Could you check a few things on this model? Use its own coordinates, in mm. A direction names the side the tool comes from. Give positions to 0.01 mm unless a question says otherwise; leave off trailing zeros. Write each loop counter-clockwise with the first axis right and the second up, starting at its lowest first coordinate (ties: lowest second). Pieces come first, ordered by that corner, then holes. Notation, with made-up numbers: M 70.5,57.5 L 129.5,57.5 A26 cw 129.5,82.5 Z; hole C -38,73.25 d11. An arc over 180 degrees is marked long. One line per item, written item: value.
```python
from build123d import *

# Parameters (mm, degrees)
SKETCH1_W                    = 482.6
SKETCH1_H                    = 381
BOSS_EXTRUDE1_DEPTH          = 0.9144
CONVERT_SOLID1_START         = -241.3
CONVERT_SOLID1_OUTLINE_W     = 0.6858
CONVERT_SOLID1_OUTLINE_H     = 381
CONVERT_SOLID1_DEPTH         = 482.6
EDGE_FLANGE1_STRIP_W         = 9.6012
EDGE_FLANGE1_STRIP_H         = 1.6002
EDGE_FLANGE1_STRIP_CUT_DEPTH = 381
EDGE_FLANGE1_DEPTH           = 381
EDGE_FLANGE2_STRIP_W         = 9.6012
EDGE_FLANGE2_STRIP_H         = 1.6002
EDGE_FLANGE2_STRIP_CUT_DEPTH = 381
EDGE_FLANGE2_DEPTH           = 381
EDGE_FLANGE3_STRIP_W         = 9.6012
EDGE_FLANGE3_STRIP_H         = 1.6002
EDGE_FLANGE3_STRIP_CUT_DEPTH = 381
EDGE_FLANGE3_DEPTH           = 381
EDGE_FLANGE4_STRIP_W         = 9.6012
EDGE_FLANGE4_STRIP_H         = 1.6002
EDGE_FLANGE4_STRIP_CUT_DEPTH = 381
EDGE_FLANGE4_DEPTH           = 381
EDGE_FLANGE5_STRIP_W         = 9.6012
EDGE_FLANGE5_STRIP_H         = 1.6002
EDGE_FLANGE5_STRIP_CUT_DEPTH = 381
EDGE_FLANGE5_DEPTH           = 381
SKETCH26_R                   = 3.2639
CUT_EXTRUDE2_DEPTH           = 2.54
SKETCH29_R                   = 3.2639
CUT_EXTRUDE4_DEPTH           = 310.870566463
SKETCH30_R                   = 3.2639
CUT_EXTRUDE5_DEPTH           = 2.54
SKETCH31_R                   = 3.19661248
CUT_EXTRUDE6_DEPTH           = 2.54
SKETCH32_R                   = 3.2639
CUT_EXTRUDE7_DEPTH           = 2.54


# Read off the part's stored shape, not the designer's step: Convert-Solid1
# Sheet-metal steps are written as plain solids
with BuildPart() as part:
    # Sketch1 → Boss-Extrude1 (new body)
    with BuildSketch(Plane(origin=(0, 0, 0), x_dir=(0, 0, -1), z_dir=(1, 0, 0))):
        Rectangle(SKETCH1_W, SKETCH1_H)
    extrude(amount=BOSS_EXTRUDE1_DEPTH)

    # Convert-Solid1 outline → Convert-Solid1 (add)
    with BuildSketch(Plane.XY.offset(CONVERT_SOLID1_START)):
        with Locations((-0.3429, 0)):
            Rectangle(CONVERT_SOLID1_OUTLINE_W, CONVERT_SOLID1_OUTLINE_H)
    extrude(amount=CONVERT_SOLID1_DEPTH)

    # Edge-Flange1 strip (across the edge) → Edge-Flange1 strip cut (cut)
    with BuildSketch(Plane(origin=(-0.6858, 190.5, -241.3), x_dir=(0, 0, 1), z_dir=(0, -1, 0))):
        with Locations((-3.2004, -0.8001)):
            Rectangle(EDGE_FLANGE1_STRIP_W, EDGE_FLANGE1_STRIP_H)
    extrude(amount=EDGE_FLANGE1_STRIP_CUT_DEPTH, mode=Mode.SUBTRACT)

    # Edge-Flange1 section (across the edge) → Edge-Flange1 (add)
    with BuildSketch(Plane(origin=(-0.6858, 190.5, -241.3), x_dir=(0, 0, 1), z_dir=(0, -1, 0))):
        with BuildLine():
            Line((-1.6002, 1.6002), (-1.6002, 23.7998))
            Line((-1.6002, 23.7998), (0, 23.7998))
            Line((0, 23.7998), (0, 1.6002))
            ThreePointArc((0, 1.6002), (0.468687729, 0.468687729), (1.6002, 0))
            Line((1.6002, 0), (1.6002, -1.6002))
            ThreePointArc((1.6002, -1.6002), (-0.662824543, -0.662824543), (-1.6002, 1.6002))
        make_face()
    extrude(amount=EDGE_FLANGE1_DEPTH)

    # Edge-Flange2 strip (across the edge) → Edge-Flange2 strip cut (cut)
    with BuildSketch(Plane(origin=(-24.4856, 190.5, -241.3), x_dir=(1, 0, 0), z_dir=(0, -1, 0))):
        with Locations((-3.2004, -0.8001)):
            Rectangle(EDGE_FLANGE2_STRIP_W, EDGE_FLANGE2_STRIP_H)
    extrude(amount=EDGE_FLANGE2_STRIP_CUT_DEPTH, mode=Mode.SUBTRACT)

    # Edge-Flange2 section (across the edge) → Edge-Flange2 (add)
    with BuildSketch(Plane(origin=(-24.4856, 190.5, -241.3), x_dir=(1, 0, 0), z_dir=(0, -1, 0))):
        with BuildLine():
            Line((-1.6002, 1.6002), (-1.6002, 23.7998))
            Line((-1.6002, 23.7998), (0, 23.7998))
            Line((0, 23.7998), (0, 1.6002))
            ThreePointArc((0, 1.6002), (0.468687729, 0.468687729), (1.6002, 0))
            Line((1.6002, 0), (1.6002, -1.6002))
            ThreePointArc((1.6002, -1.6002), (-0.662824543, -0.662824543), (-1.6002, 1.6002))
        make_face()
    extrude(amount=EDGE_FLANGE2_DEPTH)

    # Edge-Flange3 strip (across the edge) → Edge-Flange3 strip cut (cut)
    with BuildSketch(Plane(origin=(-0.6858, -190.5, 241.3), x_dir=(0, 0, -1), z_dir=(0, 1, 0))):
        with Locations((-3.2004, -0.8001)):
            Rectangle(EDGE_FLANGE3_STRIP_W, EDGE_FLANGE3_STRIP_H)
    extrude(amount=EDGE_FLANGE3_STRIP_CUT_DEPTH, mode=Mode.SUBTRACT)

    # Edge-Flange3 section (across the edge) → Edge-Flange3 (add)
    with BuildSketch(Plane(origin=(-0.6858, -190.5, 241.3), x_dir=(0, 0, -1), z_dir=(0, 1, 0))):
        with BuildLine():
            Line((-1.6002, 1.6002), (-1.6002, 23.7998))
            Line((-1.6002, 23.7998), (0, 23.7998))
            Line((0, 23.7998), (0, 1.6002))
            ThreePointArc((0, 1.6002), (0.468687729, 0.468687729), (1.6002, 0))
            Line((1.6002, 0), (1.6002, -1.6002))
            ThreePointArc((1.6002, -1.6002), (-0.662824543, -0.662824543), (-1.6002, 1.6002))
        make_face()
    extrude(amount=EDGE_FLANGE3_DEPTH)

    # Edge-Flange4 strip (across the edge) → Edge-Flange4 strip cut (cut)
    with BuildSketch(Plane(origin=(-24.4856, -190.5, 241.3), x_dir=(1, 0, 0), z_dir=(0, 1, 0))):
        with Locations((-3.2004, -0.8001)):
            Rectangle(EDGE_FLANGE4_STRIP_W, EDGE_FLANGE4_STRIP_H)
    extrude(amount=EDGE_FLANGE4_STRIP_CUT_DEPTH, mode=Mode.SUBTRACT)

    # Edge-Flange4 section (across the edge) → Edge-Flange4 (add)
    with BuildSketch(Plane(origin=(-24.4856, -190.5, 241.3), x_dir=(1, 0, 0), z_dir=(0, 1, 0))):
        with BuildLine():
            Line((-1.6002, 1.6002), (-1.6002, 23.7998))
            Line((-1.6002, 23.7998), (0, 23.7998))
            Line((0, 23.7998), (0, 1.6002))
            ThreePointArc((0, 1.6002), (0.468687729, 0.468687729), (1.6002, 0))
            Line((1.6002, 0), (1.6002, -1.6002))
            ThreePointArc((1.6002, -1.6002), (-0.662824543, -0.662824543), (-1.6002, 1.6002))
        make_face()
    extrude(amount=EDGE_FLANGE4_DEPTH)

    # Edge-Flange5 strip (across the edge) → Edge-Flange5 strip cut (cut)
    with BuildSketch(Plane(origin=(-26.0858, 190.5, 217.5002), x_dir=(0, 0, 1), z_dir=(0, -1, 0))):
        with Locations((-3.2004, -0.8001)):
            Rectangle(EDGE_FLANGE5_STRIP_W, EDGE_FLANGE5_STRIP_H)
    extrude(amount=EDGE_FLANGE5_STRIP_CUT_DEPTH, mode=Mode.SUBTRACT)

    # Edge-Flange5 section (across the edge) → Edge-Flange5 (add)
    with BuildSketch(Plane(origin=(-26.0858, 190.5, 217.5002), x_dir=(0, 0, 1), z_dir=(0, -1, 0))):
        with BuildLine():
            Line((-1.6002, 1.6002), (-1.6002, 23.7998))
            Line((-1.6002, 23.7998), (0, 23.7998))
            Line((0, 23.7998), (0, 1.6002))
            ThreePointArc((0, 1.6002), (0.468687729, 0.468687729), (1.6002, 0))
            Line((1.6002, 0), (1.6002, -1.6002))
            ThreePointArc((1.6002, -1.6002), (-0.662824543, -0.662824543), (-1.6002, 1.6002))
        make_face()
    extrude(amount=EDGE_FLANGE5_DEPTH)

    # Sketch26 → Cut-Extrude2 (cut)
    with BuildSketch(Plane(origin=(0, 0, 215.9), x_dir=(-1, 0, 0), z_dir=(0, 0, -1))):
        with Locations((39.41318, 152.4)):
            Circle(SKETCH26_R)
        with Locations((39.41318, 76.2)):
            Circle(SKETCH26_R)
        with Locations((39.41318, 0)):
            Circle(SKETCH26_R)
        with Locations((39.41318, -76.2)):
            Circle(SKETCH26_R)
        with Locations((39.41318, -152.4)):
            Circle(SKETCH26_R)
    extrude(amount=-CUT_EXTRUDE2_DEPTH, mode=Mode.SUBTRACT)

    # Sketch29 → Cut-Extrude4 (cut, through all)
    with BuildSketch(Plane.ZY.offset(26.0858)):
        with Locations((-228.6, 152.4)):
            Circle(SKETCH29_R)
        with Locations((-228.6, 76.2)):
            Circle(SKETCH29_R)
        with Locations((-228.6, 0)):
            Circle(SKETCH29_R)
        with Locations((-228.6, -76.2)):
            Circle(SKETCH29_R)
        with Locations((-228.6, -152.4)):
            Circle(SKETCH29_R)
    extrude(amount=-CUT_EXTRUDE4_DEPTH, mode=Mode.SUBTRACT)

    # Sketch30 → Cut-Extrude5 (cut)
    with BuildSketch(Plane.XY.offset(242.9002)):
        with Locations((-11.176, 152.4)):
            Circle(SKETCH30_R)
        with Locations((-11.176, 76.2)):
            Circle(SKETCH30_R)
        with Locations((-11.176, 0)):
            Circle(SKETCH30_R)
        with Locations((-11.176, -76.2)):
            Circle(SKETCH30_R)
        with Locations((-11.176, -152.4)):
            Circle(SKETCH30_R)
    extrude(amount=-CUT_EXTRUDE5_DEPTH, mode=Mode.SUBTRACT)

    # Sketch31 → Cut-Extrude6 (cut)
    with BuildSketch(Plane(origin=(0.9144, 0, 0), x_dir=(0, 0, -1), z_dir=(1, 0, 0))):
        with Locations((-217.5002, 178.689)):
            Circle(SKETCH31_R)
        with Locations((-109.5502, 178.689)):
            Circle(SKETCH31_R)
        with Locations((-1.6002, 178.689)):
            Circle(SKETCH31_R)
        with Locations((106.3498, 178.689)):
            Circle(SKETCH31_R)
        with Locations((214.2998, 178.689)):
            Circle(SKETCH31_R)
    extrude(amount=-CUT_EXTRUDE6_DEPTH, mode=Mode.SUBTRACT)

    # Sketch32 → Cut-Extrude7 (cut)
    with BuildSketch(Plane.ZY.offset(0.6858)):
        with Locations((-214.2998, -178.7144)):
            Circle(SKETCH32_R)
        with Locations((-112.6998, -178.7144)):
            Circle(SKETCH32_R)
        with Locations((-11.0998, -178.7144)):
            Circle(SKETCH32_R)
        with Locations((90.5002, -178.7144)):
            Circle(SKETCH32_R)
        with Locations((192.1002, -178.7144)):
            Circle(SKETCH32_R)
    extrude(amount=-CUT_EXTRUDE7_DEPTH, mode=Mode.SUBTRACT)


solid = part.part
```
1) If we section it at A-A, the plane y = 65: Write out the boundary of the cut face in (x, z).
Outcome:
outline: M -49.89,215.9 L -27.69,215.9 A3.2 ccw -24.49,219.1 L -24.49,239.7 A1.6 cw -22.89,241.3 L -2.29,241.3 A1.6 cw -0.69,239.7 L -0.69,-239.7 A1.6 cw -2.29,-241.3 L -22.89,-241.3 A1.6 cw -24.49,-239.7 L -24.49,-217.5 L -26.09,-217.5 L -26.09,-239.7 A3.2 ccw -22.89,-242.9 L -2.29,-242.9 A3.2 ccw 0.91,-239.7 L 0.91,239.7 A3.2 ccw -2.29,242.9 L -22.89,242.9 A3.2 ccw -26.09,239.7 L -26.09,219.1 A1.6 cw -27.69,217.5 L -49.89,217.5 Z
2) On a 3-axis mill with a long thin cutter (end or side, diameter ignored), from which of +Z, -Z, +X, -X, +Y, -Y can I reach the whole of each face in a straight line? I mean faces 1 (the face through (-12, 3, -242.9)), 2 (the face through (-26.086, -3, 230)), 3 (the face through (-26.086, 3, -231)), 4 (the face through (-13, 3, -241.3)), 5 (the face through (0, -190.5, 73)). Say none if no direction works.
Outcome:
face 1: -Z, +X, -X, +Y, -Y
face 2: +Z, -X, +Y, -Y
face 3: -Z, -X, +Y, -Y
face 4: +Y, -Y
face 5: +Z, -Z, +X, -X, -Y
3) I'm going to push flat-ended pins straight in: pin 1 (7.5 mm diameter, centred on x = -39.41, y = 152.4, fed in from -Z); pin 2 (10.5 mm diameter, centred on y = 0, z = -228.6, fed in from -X); pin 3 (7.5 mm diameter, centred on y = 178.69, z = 1.6, fed in from -X). Where does each tip first touch, or does it pass through?
Outcome:
pin 1: stops at z = 215.9
pin 2: stops at x = -26.09
pin 3: stops at x = -0.69
4) We'd pull the mould along Z, two halves only. Please class faces 6 (the face through (-0.686, -3, -3)), 7 (the face through (-15, -3, 242.9)), 8 (the face through (0, 190.5, 73)), 9 (the face through (-15, -3, 241.3)): pulls with the +Z half, pulls with the -Z half, needs draft (parallel to the pull), parting line crosses it, or undercut.
Outcome:
face 6: undercut
face 7: pulls with the +Z half
face 8: needs draft
face 9: undercut
5) If we section it at B-B, the plane z = -198: Write out the boundary of the cut face in (x, y), then the cut area to 3 significant figures.
Outcome:
outline: M -0.69,-190.5 L 0.91,-190.5 L 0.91,190.5 L -0.69,190.5 Z
area: 610 mm^2
6) Please list where these lines run through material, in increasing order: L1, parallel to Y at x = 0, z = -228; L2, parallel to Z at x = -22, y = -96; L3, parallel to Z at x = -37.5, y = -126.5. Write a range as from..to.
Outcome:
L1: y = -190.5..-155.61, -149.19..-79.41, -72.99..-3.21, 3.21..72.99, 79.41..149.19, 155.61..190.5
L2: z = -242.9..-241.3, 241.3..242.9
L3: z = 215.9..217.5
